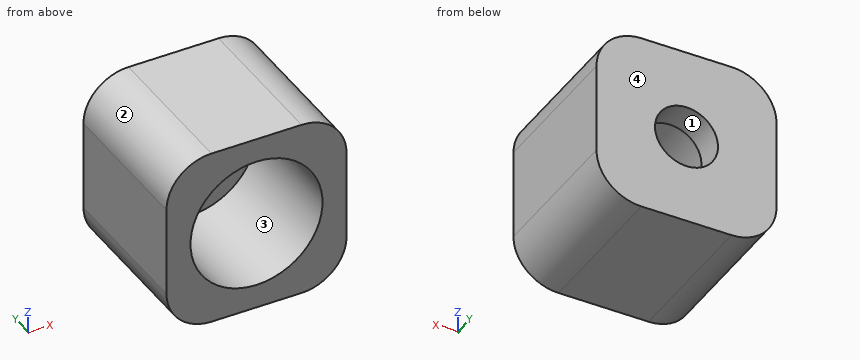
```python
from build123d import *

# Parameters (mm, degrees)
SKETCH1_R           = 2.1
BOSS_EXTRUDE1_DEPTH = 10
SKETCH2_R           = 4.4
CUT_EXTRUDE1_DEPTH  = 8


with BuildPart() as part:
    # Sketch1 → Boss-Extrude1 (new body)
    with BuildSketch(Plane(origin=(0, 0, 0), x_dir=(1, 0, 0), z_dir=(0, 1, 0))):
        with BuildLine():
            Line((-3, -6), (3, -6))
            ThreePointArc((3, -6), (5.121320344, -5.121320344), (6, -3))
            Line((6, -3), (6, 3))
            ThreePointArc((6, 3), (5.121320344, 5.121320344), (3, 6))
            Line((3, 6), (-3, 6))
            ThreePointArc((-3, 6), (-5.121320344, 5.121320344), (-6, 3))
            Line((-6, 3), (-6, -3))
            ThreePointArc((-6, -3), (-5.121320344, -5.121320344), (-3, -6))
        make_face()
        with Locations(Location((0, 0, 0), (0, 0, 270))):
            Circle(SKETCH1_R, mode=Mode.SUBTRACT)
    extrude(amount=BOSS_EXTRUDE1_DEPTH)

    # Sketch2 → Cut-Extrude1 (cut)
    with BuildSketch(Plane.XZ):
        with Locations(Location((0, 0, 0), (0, 0, 270))):
            Circle(SKETCH2_R)
    extrude(amount=-CUT_EXTRUDE1_DEPTH, mode=Mode.SUBTRACT)


solid = part.part
```
Design review of the part built by this model. Coordinates are the model's own, in mm. Face numbers are marked on the shaded views. Coordinates: 2 decimals unless noted, no trailing zeros. Order: outer loops, then holes, each group sorted by start corner. A loop starts at its lowest first (then second) coordinate and runs counter-clockwise, first axis right, second up. Notation, with made-up numbers: (-26.75, 62) -> (-8.75, 62) arc R18 ccw to (-8.75, 84) -> close; hole circle Ø10 at (61, -14). An arc over 180 degrees is marked (long way). One line per item, written item: value. Start each with the question number.
Q1. Take a section at C-C, the plane y = 9. State the section outline as (x, z) points, then the cut area to 3 significant figures.
Q2. Take a section at B-B, the plane z = 0. State the section outline as (x, y) points.
Q3. Insertion check: pin 1 Ø6 at (x, y) = (3.5, 9) entering from -Z; pin 2 Ø2.5 at (x, z) = (-1.5, 0) entering from -Y; pin 3 Ø2 at (y, z) = (2.5, 4.5) entering from -X. Each pin has a flat end and moves straight along its axis. Give the tip position at first contact, or say it passes through.
Q4. For probe 1 along X at (y, z) = (9.1, 0); probe 2 along X at (y, z) = (3.25, 0), list the stretches that pass through material, from the lowest coordinate up.
Q5. Take a section at A-A, the plane x = 0. State the section outline as (y, z) points, then the cut area to 3 significant figures.
Q6. Take a section at D-D, the plane x = -3.75. State the section outline as (y, z) points.
Q7. Mouldability with a two-part tool opening along Z and no side actions: class the marked faces 1, 2, 3 and 4 as pulls with the +Z half, pulls with the -Z half, needs draft (parallel to the pull), parting line crosses it, or undercut.
Values follow:
1. outline: (-6, -3) arc R3 ccw to (-3, -6) -> (3, -6) arc R3 ccw to (6, -3) -> (6, 3) arc R3 ccw to (3, 6) -> (-3, 6) arc R3 ccw to (-6, 3) -> close; hole circle Ø4.2 at (0, 0)
1. area: 122 mm2
2. outline: (-6, 0) -> (-4.4, 0) -> (-4.4, 8) -> (-2.1, 8) -> (-2.1, 10) -> (-6, 10) -> close; (2.1, 8) -> (4.4, 8) -> (4.4, 0) -> (6, 0) -> (6, 10) -> (2.1, 10) -> close
3. pin 1: stops at z = -6
3. pin 2: stops at y = 8
3. pin 3: stops at x = -5.96
4. probe 1: x = -6 to -2.1, 2.1 to 6
4. probe 2: x = -6 to -4.4, 4.4 to 6
5. outline: (0, -6) -> (10, -6) -> (10, -2.1) -> (8, -2.1) -> (8, -4.4) -> (0, -4.4) -> close; (0, 4.4) -> (8, 4.4) -> (8, 2.1) -> (10, 2.1) -> (10, 6) -> (0, 6) -> close
5. area: 41.2 mm2
6. outline: (0, -5.9) -> (10, -5.9) -> (10, 5.9) -> (0, 5.9) -> (0, 2.3) -> (8, 2.3) -> (8, -2.3) -> (0, -2.3) -> close
7. face 1: undercut
7. face 2: pulls with the +Z half
7. face 3: undercut
7. face 4: needs draft
